Solid Edge part; units mm, degrees
sketch "Sketch1" plane through (0, 0, 0) normal (0, -1, 0) x (1, 0, 0)
  line L0 (-12, 9) -> (12, 9)
  line L1 (12, 9) -> (12, -16)
  line L2 (10, -16) -> (12, -16)
  line L3 (10, -16) -> (10, 6)
  line L4 (10, 6) -> (-10, 6)
  line L5 (-10, 6) -> (-10, -16)
  line L6 (-12, -16) -> (-10, -16)
  line L7 (-12, -16) -> (-12, 9)
extrude "Protrusion1" add sketch "Sketch1" along normal mid plane 10
sketch "Sketch2" plane through (-10, 0, -5) normal (1, 0, 0) x (0, 1, 0)
  circle A0 centre (0, -7.0612) radius 2
extrude "ExtrudedProtrusion_5" add sketch "Sketch2" along normal blind 20
sketch "Sketch3" plane through (0, 0, 9) normal (0, 0, 1) x (1, 0, 0)
  line L0 (2.5, -1.5) -> (2.5, 1.5)
  line L1 (2.5, 1.5) -> (-2.5, 1.5)
  line L2 (-2.5, 1.5) -> (-2.5, -1.5)
  line L3 (-2.5, -1.5) -> (2.5, -1.5)
extrude "ExtrudedProtrusion_6" add sketch "Sketch3" along normal blind 50
sketch "Sketch4" plane through (0, -1.5, 34) normal (0, -1, 0) x (0, 0, 1)
  circle A0 centre (21.4608, 0.0773) radius 3.5
extrude "ExtrudedProtrusion_9" add sketch "Sketch4" against normal blind 17 and the other way blind 12
sketch "Sketch5" plane through (-0.0773, -13.5, 55.4608) normal (0, -1, 0) x (0, 0, 1)
  circle A0 centre (0.0243, -0.0243) radius 2.5
extrude "ExtrudedCutout_2" cut sketch "Sketch5" against normal blind 47.3814
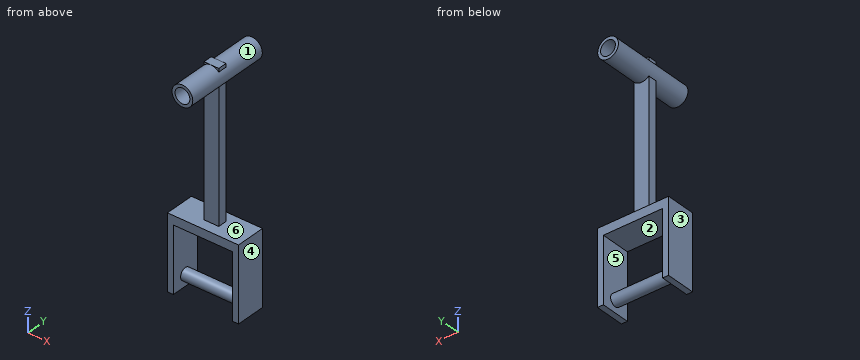
Work out the finished part from the listing and answer in its coordinate system (mm). Face numbers are marked on the shaded views. A direction names the side the tool comes from. Round coordinates to 2 decimals unless told otherwise and drop trailing zeros. Write each loop counter-clockwise with the first axis right and the second up, starting at its lowest first coordinate (ties: lowest second). Pieces come first, ordered by that corner, then holes. Notation, with made-up numbers: (-29.5, -37.5) - (-6.5, -37.5) arc R22 cw to (-6.5, -2.5) - close; hole circle Ø9 at (71, 36.25). An arc over 180 degrees is marked (long way). Return JSON: item names as keys, results as strings. Group by question number.
Q1. The part is cut by section D-D on y = -6.75. Write down the section's boundary in (x, z), then the cut area to 3 significant figures.
Q2. Each of these flat-tipped pins is pushed along its axis until it touches: pin 1 Ø5.5 at (x, z) = (-0.5, 39) entering from +Y; pin 2 Ø0.6 at (y, z) = (0.5, 58.5) entering from +X; pin 3 Ø10 at (x, y) = (0, 8.5) entering from +Z. Where does it stop, or does it pass through?
Q3. The part is cut by section A-A on z = -3. Write down the section's boundary in (x, y).
Q4. The mould has two halves that part along X. Classify the marked faces 4, 5 and 6: released by +X, released by -X, zero draft, split by the parting line, or undercut.
Q5. For the marked faces 1, 2 and 3, determine the directions among +Z, -Z, +X, -X, +Y, -Y from which every point of the face is accessible in a straight line to the end or side of a thin tool.
Q6. The part is cut by section B-B on x = -7.25. Write down the section's boundary in (y, z).
Q7. Find the intervals of material crossed by L1, parallel to Z at x = 0, y = -6; L2, parallel to X at y = 2.5, z = -3.5; L3, parallel to Y at x = -10.75, z = 8.5, in increasing order.
Q8. The part is cut by section C-C on y = 0. Write down the section's boundary in (x, z).
Solved:
{
 "1": {"outline": "circle Ø7 at (-0.08, 55.46); hole circle Ø5 at (-0.05, 55.49)", "area": "18.8 mm²"},
 "2": {"pin 1": "y = 1.5", "pin 2": "x = 2.5", "pin 3": "z = 58.96"},
 "3": {"outline": "(-12, -5) - (-10, -5) - (-10, 5) - (-12, 5) - close; (10, -5) - (12, -5) - (12, 5) - (10, 5) - close"},
 "4": {"face 4": "released by +X", "face 5": "undercut", "face 6": "zero draft"},
 "5": {"face 1": "none", "face 2": "+Y, -Y", "face 3": "+Z, -Z, -X, +Y, -Y"},
 "6": {"outline": "(-5, 6) - (5, 6) - (5, 9) - (-5, 9) - close; circle Ø4 at (0, -12.06)"},
 "7": {"L1": "51.96 to 52.99, 57.98 to 58.96", "L2": "-12 to -10, 10 to 12", "L3": "-5 to 5"},
 "8": {"outline": "(-12, -16) - (-10, -16) - (-10, -14.06) - (10, -14.06) - (10, -16) - (12, -16) - (12, 9) - (2.5, 9) - (2.5, 53.09) arc R3.5 ccw to (2.5, 57.83) - (2.5, 59) - (-2.5, 59) - (-2.5, 57.99) arc R3.5 ccw to (-2.5, 52.93) - (-2.5, 9) - (-12, 9) - close; hole (-10, -10.06) - (10, -10.06) - (10, 6) - (-10, 6) - close; hole circle Ø5 at (-0.05, 55.49)"}
}
